Geometry: final body of the model. Coordinates: model frame, mm. Face numbers are marked on the shaded views. A direction names the side the tool comes from. Give positions to 0.01 mm unless a question says otherwise; leave off trailing zeros. Write each loop counter-clockwise with the first axis right and the second up, starting at its lowest first coordinate (ties: lowest second). Pieces come first, ordered by that corner, then holes.
from build123d import *

# Parameters (mm, degrees)
F0_R      = 29.6723424489
F1_DEPTH  = 38.1
F2_DEPTH  = 38.1
F3_DEPTH  = 76.2
F4_W      = 59.6218928695
F4_H      = 20.4950273037
F5_DEPTH  = 50.8
F6_DEPTH  = 50.8
F8_DEPTH  = 19.558
F10_DEPTH = 19.05
F12_DEPTH = 18.796
F13_R     = 15.1650839795
F14_DEPTH = 203.2
F15_R     = 15.8233600447
F16_DEPTH = 177.8


with BuildPart() as f1:
    # F0 (on Front) → F1 (new body)
    with BuildSketch(Plane.XZ):
        with Locations((0, -51.4704622328)):
            Circle(F0_R)
    extrude(amount=F1_DEPTH)

    # F2 (add): a face of the model
    f2_faces = [f1.faces().sort_by_distance(p)[0] for p in [
        (0, -38.1, -51.4704622328),
    ]]
    extrude(f2_faces, amount=F2_DEPTH)

    # F3 (add): a face of the model
    f3_faces = [f1.faces().sort_by_distance(p)[0] for p in [
        (0, 0, -51.4704622328),
    ]]
    extrude(f3_faces, amount=F3_DEPTH)

    # F4 (on Top) → F5 (join)
    with BuildSketch(Plane.XY):
        with Locations((1.8626e-06, -65.9101381898)):
            Rectangle(F4_W, F4_H)
    extrude(amount=-F5_DEPTH)

    # F6 (add): a face of the model
    f6_faces = [f1.faces().sort_by_distance(p)[0] for p in [
        (1.8626e-06, -65.9101381898, 0),
    ]]
    extrude(f6_faces, amount=F6_DEPTH)

    # F7 (on face) → F8 (join)
    with BuildSketch(Plane.XZ.offset(76.1576518416)):
        with BuildLine():
            Line((-29.2987728327, 50.8), (29.298776558, 50.8))
            ThreePointArc((29.298776558, 50.8), (1.8626e-06, 80.0987746954), (-29.2987728327, 50.8))
        make_face()
    extrude(amount=-F8_DEPTH)

    # F9 (on face) → F10 (join)
    with BuildSketch(Plane(origin=(0, 76.2, 0), x_dir=(-1, 0, 0), z_dir=(0, 1, 0))):
        with BuildLine():
            Line((-29.6259251728, 51.0046631098), (-29.6259251728, -49.811407061))
            ThreePointArc((-29.6259251728, -49.811407061), (-1.3748108286, -21.8299865013), (29.3451528996, -47.0761582262))
            Line((29.3451528996, -47.0761582262), (29.3451528996, 51.0046631098))
            Line((29.3451528996, 51.0046631098), (-29.6259251728, 51.0046631098))
        make_face()
    extrude(amount=-F10_DEPTH)

    # F11 (on face) → F12 (join)
    with BuildSketch(Plane(origin=(0, 76.2, 0), x_dir=(-1, 0, 0), z_dir=(0, 1, 0))):
        with BuildLine():
            Line((-29.4398787195, 51.0046631098), (29.1591064463, 51.0046631098))
            ThreePointArc((29.1591064463, 51.0046631098), (-0.1403861366, 80.3041556927), (-29.4398787195, 51.0046631098))
        make_face()
    extrude(amount=-F12_DEPTH)

    # F13 (on face) → F14 (cut)
    with BuildSketch(Plane(origin=(0, 76.2, 0), x_dir=(-1, 0, 0), z_dir=(0, 1, 0))):
        with Locations((0, -49.811407061)):
            Circle(F13_R)
    extrude(amount=-F14_DEPTH, mode=Mode.SUBTRACT)

    # F15 (on face) → F16 (cut)
    with BuildSketch(Plane(origin=(0, 76.2, 0), x_dir=(-1, 0, 0), z_dir=(0, 1, 0))):
        with Locations((0, 51.0046631098)):
            Circle(F15_R)
    extrude(amount=-F16_DEPTH, mode=Mode.SUBTRACT)


solid = f1.part
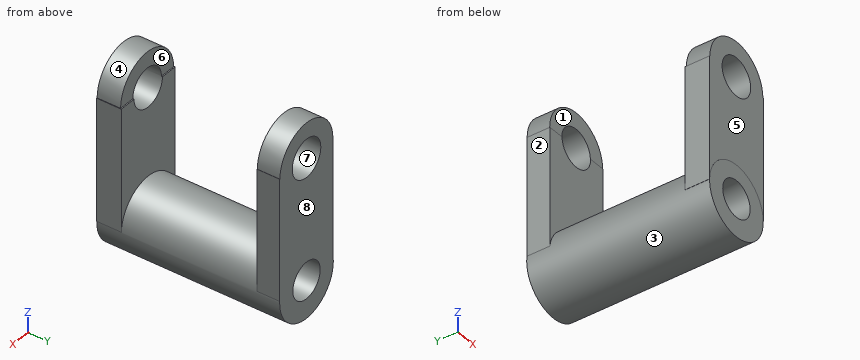
Q1. Section A-A on z = -1. Output: boundary loops of the cut face in (x, y).
Filled sheet:
outline: (-29.81, -76.16) - (29.81, -76.16) - (29.81, -55.66) - (-29.81, -55.66) - close; (-29.35, 57.15) - (29.63, 57.15) - (29.63, 76.2) - (-29.35, 76.2) - close
Q2. Pin query (flat end, axial travel): P1, Ø1, axis at x = 17, y = 30.5, coming from the +Z side; P2, Ø10, axis at x = 19, y = -56.5, coming from the +Z side; P3, Ø9.5, axis at y = 67.5, z = -2, coming from the +X side; P4, Ø4, axis at x = 7.5, z = -61, coming from the +Y side. Return the tip coordinate at first contact, or that it passes through.
Filled sheet:
P1: stops at z = -26.81
P2: stops at z = 76.54
P3: stops at x = 29.63
P4: stops at y = 76.2
Q3. Access query for the marked faces 1, 2, 3 and 4. Directions: +Z, -Z, +X, -X, +Y, -Y. A direction counts if a zero-diameter tool reaches every point of the face in a straight line with its end or side. Return the directions, or none.
Filled sheet:
face 1: +Z, +X, -X
face 2: +Z, -X, +Y
face 3: none
face 4: +Z, -Y
Q4. Section B-B on x = 0. Output: boundary loops of the cut face in (y, z), plus the area to 3 significant figures.
Filled sheet:
outline: (-76.2, -81.14) - (76.2, -81.14) - (76.2, -64.98) - (-76.2, -64.98) - close; (-76.2, -34.65) - (76.2, -34.65) - (76.2, 35.18) - (57.15, 35.18) - (57.15, -21.8) - (-55.66, -21.8) - (-55.66, 35.18) - (-76.16, 35.18) - (-76.16, -21.8) - (-76.2, -21.8) - close; (-76.16, 66.83) - (-56.6, 66.83) - (-56.6, 80.1) - (-76.16, 80.1) - close; (57.4, 66.83) - (76.2, 66.83) - (76.2, 80.3) - (57.4, 80.3) - close
area: 7,190 mm2
Q5. Pull-direction query (Y, two-part tool) for the marked faces 5, 6, 7 and 8; classes: released by +Y, released by -Y, zero draft, split by the parting line, or undercut.
Filled sheet:
face 5: released by -Y
face 6: undercut
face 7: zero draft
face 8: released by +Y
Q6. Section C-C on y = -61. Output: boundary loops of the cut face in (x, z), plus the area to 3 significant figures.
Filled sheet:
outline: (-29.81, -50.8) - (-29.66, -50.8) arc R29.67 ccw (long way) to (29.66, -50.8) - (29.81, -50.8) - (29.81, 50.8) - (29.3, 50.8) arc R29.3 ccw to (-29.3, 50.8) - (-29.81, 50.8) - close; hole circle Ø31.65 at (0, 51); hole circle Ø30.33 at (0, -49.81)
area: 7,320 mm2
Q7. Ray query, line 1 along Z through (x, y) = (0, 71.75); line 2 along Z through (x, y) = (0, -67); line 3 along Y through (x, z) = (-16.5, 72). Return the intervals inside material, ascending.
Filled sheet:
line 1: z = -81.14 to -64.98, -34.65 to 35.18, 66.83 to 80.3
line 2: z = -81.14 to -64.98, -34.65 to 35.18, 66.83 to 80.1
line 3: y = -76.16 to -56.6, 57.4 to 76.2
Q8. Section D-D on z = 53. Output: boundary loops of the cut face in (x, y).
Filled sheet:
outline: (-29.22, -76.16) - (-15.7, -76.16) - (-15.7, -56.6) - (-29.22, -56.6) - close; (-29.09, 57.4) - (-15.7, 57.4) - (-15.7, 76.2) - (-29.09, 76.2) - close; (15.7, -76.16) - (29.22, -76.16) - (29.22, -56.6) - (15.7, -56.6) - close; (15.7, 57.4) - (29.37, 57.4) - (29.37, 76.2) - (15.7, 76.2) - close
